from build123d import *

# Parameters (mm, degrees)
F0_R         = 31
F1_DEPTH     = 10
F2_R         = 2.35
F3_DEPTH     = 22.7863546661
F6_T1_DEPTH  = 14.0295669578
F6_T4_ANGLE  = 314.9633717383
F6_T6_ANGLE  = 314.9633717383
F6_T12_ANGLE = 67.4816858691
F6_T14_ANGLE = 67.4816858691
F6_T16_ANGLE = 67.4816858691
F6_T18_ANGLE = 67.4816858691


# Not quite as in the source:
# - a fillet or chamfer that OpenCascade refuses, or shapes differently, is made with other operations: its cross-section is extruded or revolved along the edge and cut away or added


with BuildPart() as f1:
    # F0 (on Top) → F1 (new body)
    with BuildSketch(Plane.XY):
        with BuildLine():
            ThreePointArc((-10, 43.4165866922), (-11.3475328525, 38.9730879748), (-14.9361702128, 36.0265293829))
            ThreePointArc((-14.9361702128, 36.0265293829), (0, -39), (14.9361702128, 36.0265293829))
            ThreePointArc((14.9361702128, 36.0265293829), (11.3475328525, 38.9730879748), (10, 43.4165866922))
            Line((10, 43.4165866922), (10, 53.6961536499))
            Line((10, 53.6961536499), (-10, 53.6961536499))
            Line((-10, 53.6961536499), (-10, 43.4165866922))
        make_face()
        Circle(F0_R, mode=Mode.SUBTRACT)
    extrude(amount=F1_DEPTH)

    # F2 (on face) → F3 (cut, through all)
    with BuildSketch(Plane(origin=(0, 53.6961536499, 0), x_dir=(-1, 0, 0), z_dir=(0, 1, 0))):
        with Locations((0, 5)):
            Circle(F2_R)
    extrude(amount=-F3_DEPTH, mode=Mode.SUBTRACT)

    # F4 (on Right) → F5 (revolve, cut)
    with BuildSketch(Plane.YZ):
        Polygon((35.1961536499, 5), (30.1961536499, 10), (30.1961536499, 5), align=None)
    revolve(axis=Axis((0, 32.6961536499, 5), (0, -1, 0)), mode=Mode.SUBTRACT)

    # F6: fillet of radius 1.5 on 12 edges, made by hand

    # F6_s2 → F6_t1 (cut)
    with BuildSketch(Plane.XZ.offset(-57.4461536499)):
        with BuildLine():
            ThreePointArc((-10, 1.5), (-9.5606601718, 0.4393398282), (-8.5, 0))
            Line((-8.5, 0), (-10, 0))
            Line((-10, 0), (-10, 1.5))
        make_face()
        with BuildLine():
            ThreePointArc((-10, 8.5), (-9.5606601718, 9.5606601718), (-8.5, 10))
            Line((-8.5, 10), (-10, 10))
            Line((-10, 10), (-10, 8.5))
        make_face()
        with BuildLine():
            ThreePointArc((8.5, 0), (9.5606601718, 0.4393398282), (10, 1.5))
            Line((10, 1.5), (10, 0))
            Line((10, 0), (8.5, 0))
        make_face()
        with BuildLine():
            ThreePointArc((8.5, 10), (9.5606601718, 9.5606601718), (10, 8.5))
            Line((10, 8.5), (10, 10))
            Line((10, 10), (8.5, 10))
        make_face()
    extrude(amount=F6_T1_DEPTH, mode=Mode.SUBTRACT)

    # F6_s3 → F6_t4 (revolve, cut)
    with BuildSketch(Plane(origin=(0, 0, 0), x_dir=(0, 0, 1), z_dir=(0.9237571637, 0.3829787234, 0))):
        with BuildLine():
            ThreePointArc((8.5, -39), (9.5606601718, -38.5606601718), (10, -37.5))
            Line((10, -37.5), (10, -39))
            Line((10, -39), (8.5, -39))
        make_face()
    revolve(axis=Axis((0, 0, 10), (0, 0, 1)), revolution_arc=F6_T4_ANGLE, mode=Mode.SUBTRACT)

    # F6_s5 → F6_t6 (revolve, cut)
    with BuildSketch(Plane(origin=(0, 0, 0), x_dir=(0, 0, 1), z_dir=(0.9237571637, 0.3829787234, 0))):
        with BuildLine():
            ThreePointArc((1.5, -39), (0.4393398282, -38.5606601718), (0, -37.5))
            Line((0, -37.5), (0, -39))
            Line((0, -39), (1.5, -39))
        make_face()
    revolve(axis=Axis((0, 0, 0), (0, 0, 1)), revolution_arc=F6_T6_ANGLE, mode=Mode.SUBTRACT)

    # F6_s7 → F6_t8 (revolve, cut)
    with BuildSketch(Plane.XZ):
        with BuildLine():
            ThreePointArc((32.5, 0), (31.4393398282, 0.4393398282), (31, 1.5))
            Line((31, 1.5), (31, 0))
            Line((31, 0), (32.5, 0))
        make_face()
    revolve(axis=Axis((0, 0, 0), (0, 0, 1)), mode=Mode.SUBTRACT)

    # F6_s9 → F6_t10 (revolve, cut)
    with BuildSketch(Plane.XZ):
        with BuildLine():
            ThreePointArc((32.5, 10), (31.4393398282, 9.5606601718), (31, 8.5))
            Line((31, 8.5), (31, 10))
            Line((31, 10), (32.5, 10))
        make_face()
    revolve(axis=Axis((0, 0, 10), (0, 0, 1)), mode=Mode.SUBTRACT)

    # F6_s11 → F6_t12 (revolve, cut)
    with BuildSketch(Plane.XZ.offset(-43.4165866922)):
        with BuildLine():
            ThreePointArc((-10, 1.5), (-9.5606601718, 0.4393398282), (-8.5, 0))
            Line((-8.5, 0), (-10, 0))
            Line((-10, 0), (-10, 1.5))
        make_face()
    revolve(axis=Axis((-18, 43.4165866922, 0), (0, 0, -1)), revolution_arc=F6_T12_ANGLE, mode=Mode.SUBTRACT)

    # F6_s13 → F6_t14 (revolve, cut)
    with BuildSketch(Plane.XZ.offset(-43.4165866922)):
        with BuildLine():
            ThreePointArc((-10, 8.5), (-9.5606601718, 9.5606601718), (-8.5, 10))
            Line((-8.5, 10), (-10, 10))
            Line((-10, 10), (-10, 8.5))
        make_face()
    revolve(axis=Axis((-18, 43.4165866922, 10), (0, 0, -1)), revolution_arc=F6_T14_ANGLE, mode=Mode.SUBTRACT)

    # F6_s15 → F6_t16 (revolve, cut)
    with BuildSketch(Plane(origin=(0, 0, 0), x_dir=(0, 0, 1), z_dir=(0.9237571637, -0.3829787234, 0))):
        with BuildLine():
            ThreePointArc((0, -37.5), (0.4393398282, -38.5606601718), (1.5, -39))
            Line((1.5, -39), (0, -39))
            Line((0, -39), (0, -37.5))
        make_face()
    revolve(axis=Axis((18, 43.4165866922, 0), (0, 0, -1)), revolution_arc=F6_T16_ANGLE, mode=Mode.SUBTRACT)

    # F6_s17 → F6_t18 (revolve, cut)
    with BuildSketch(Plane(origin=(0, 0, 0), x_dir=(0, 0, 1), z_dir=(0.9237571637, -0.3829787234, 0))):
        with BuildLine():
            ThreePointArc((10, -37.5), (9.5606601718, -38.5606601718), (8.5, -39))
            Line((8.5, -39), (10, -39))
            Line((10, -39), (10, -37.5))
        make_face()
    revolve(axis=Axis((18, 43.4165866922, 10), (0, 0, -1)), revolution_arc=F6_T18_ANGLE, mode=Mode.SUBTRACT)


solid = f1.part
Geometry: final body of the model. Coordinates: model frame, mm. A direction names the side the tool comes from. Give positions to 0.01 mm unless a question says otherwise; leave off trailing zeros. Write each loop counter-clockwise with the first axis right and the second up, starting at its lowest first coordinate (ties: lowest second). Pieces come first, ordered by that corner, then holes. Notation, with made-up numbers: M -16.5,77 L 12.5,77 A17 ccw 12.5,95 Z; hole C 55.25,79.5 d2. An arc over 180 degrees is marked long. Answer in a Markdown table with one row per item. Add a question column.
(1) Section C-C on x = 0. Return loops of the section in (y, z).
(2) First-contact query: pin 1 (1 mm diameter, centred on x = -28.5, z = 7.5, fed in from -Y); pin 2 (3.5 mm diameter, centred on y = 50, z = 4, fed in from -X); pin 3 (2 mm diameter, centred on y = 50.5, z = 6.5, fed in from +X); pin 4 (5.5 mm diameter, centred on x = 0, z = 5, fed in from +Y). Flat tips, straight axial feed; report the tip coordinate or a pass-through.
(3) Section B-B on z = 5. Return loops of the section in (x, y).
(4) Mould query, pull axis Z, two halves, no side actions, for faces 1 (the conical face through (2.427, 32.71, 4.461)), 2 (the flat face through (8, 32, 0)), 3 (the flat face through (8, 32, 10)), 4 (the cylindrical face through (-11.31, 39.03, 4.95)). Classes: +Z half, -Z half, draft (parallel to the pull), parting line (faces both ways), or undercut.
(5) Ray query, line 1 (Z direction, x = 0, y = 38.25); line 2 (X direction, y = 0, z = 5); line 3 (Y direction, x = 0, z = 5.5). Return the intervals inside material, ascending.
(6) Reachability of faces 5 (the flat face through (10, 48, 5)), 6 (the cylindrical face through (0.509, 43.417, 2.706)), 7 (the flat face through (-10, 49, 5)) from +Z, -Z, +X, -X, +Y, -Y: full face, straight path, thin tool, end or side. Return the list, or none.
(7) Section A-A on y = 0. Return loops of the section in (x, z).
Result set:
| question | item | result |
|---|---|---|
| 1 | outline | M -39,1.5 A1.5 ccw -37.5,0 L -32.5,0 A1.5 ccw -31,1.5 L -31,8.5 A1.5 ccw -32.5,10 L -37.5,10 A1.5 ccw -39,8.5 Z; M 31.12,0.92 A1.5 ccw 32.5,0 L 53.7,0 L 53.7,2.65 L 32.85,2.65 Z; M 31.12,9.08 L 32.85,7.35 L 53.7,7.35 L 53.7,10 L 32.5,10 A1.5 ccw Z |
| 2 | pin 1 | stops at y = -27.15 |
| 2 | pin 2 | stops at x = -10 |
| 2 | pin 3 | stops at x = 10 |
| 2 | pin 4 | stops at y = 53.7 |
| 3 | outline | M -14.94,36.03 A39 ccw long 14.94,36.03 A8 cw 10,43.42 L 10,53.7 L 2.35,53.7 L 2.35,32.85 L 4.53,30.67 A31 cw long -4.53,30.67 L -2.35,32.85 L -2.35,53.7 L -10,53.7 L -10,43.42 A8 cw Z |
| 4 | face 1 | undercut |
| 4 | face 2 | -Z half |
| 4 | face 3 | +Z half |
| 4 | face 4 | draft |
| 5 | line 1 | z = 0 to 2.65, 7.35 to 10 |
| 5 | line 2 | x = -39 to -31, 31 to 39 |
| 5 | line 3 | y = -39 to -31 |
| 6 | face 5 | +Z, -Z, +X, +Y |
| 6 | face 6 | +Y |
| 6 | face 7 | +Z, -Z, -X, +Y |
| 7 | outline | M -39,1.5 A1.5 ccw -37.5,0 L -32.5,0 A1.5 ccw -31,1.5 L -31,8.5 A1.5 ccw -32.5,10 L -37.5,10 A1.5 ccw -39,8.5 Z; M 31,1.5 A1.5 ccw 32.5,0 L 37.5,0 A1.5 ccw 39,1.5 L 39,8.5 A1.5 ccw 37.5,10 L 32.5,10 A1.5 ccw 31,8.5 Z |
